Input: part model. Units: mm. Frame: model coordinates. Face numbers are marked on the shaded views. A direction names the side the tool comes from. Give positions to 0.01 mm unless a question says otherwise; leave off trailing zeros. Loops run counter-clockwise (first coordinate to the right, second up) from the corner with the lowest first, then second, coordinate; pieces in that order, holes last. Notation, with made-up numbers: (-32.75, -12) - (1.25, -12) arc R17 ccw to (1.25, 0) - close; hole circle Ø9 at (41, 24). An arc over 180 degrees is marked (long way). Answer as a JSON object with one key per item and string values. Group by question number.
(1) Access query for the marked faces 1, 2 and 3. Directions: +Z, -Z, +X, -X, +Y, -Y. A direction counts if a zero-diameter tool reaches every point of the face in a straight line with its end or side. Return the directions, or none.
(2) Material intervals for L1, parallel to Y at x = 0, z = 13; L2, parallel to Z at x = 12.5, y = 2; L3, parallel to Y at x = 8, z = 184.5, sorted ascending.
(3) Section query A-A (z = 174.5). Return loops of the section in (x, y), plus the area to 3 significant figures.
(4) Section query B-B (z = 126). Return loops of the section in (x, y).
(5) Pin query (flat end, axial travel): P1, Ø5, axis at x = 8.5, z = 166, coming from the -Y side; P2, Ø9.5, axis at x = 0, y = 0, coming from the +Z side; P3, Ø5, axis at y = 7, z = 63, coming from the +X side. Return the tip coordinate at first contact, or that it passes through.
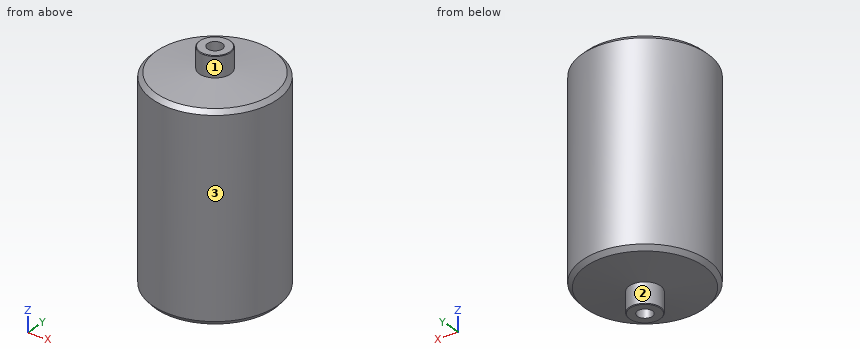
```python
from build123d import *
from OCP.BRepFilletAPI import BRepFilletAPI_MakeChamfer

# Parameters (mm, degrees)
CHAFL_N1_SIZE                     = 3
CHAFL_N1_SIZE2                    = 3.300188603
TALADRO_DE_MARGEN_PARA_M101_D     = 12
TALADRO_DE_MARGEN_PARA_M101_DEPTH = 55.394836286
TALADRO_DE_MARGEN_PARA_M101_TIP   = 3.605163714
TALADRO_DE_MARGEN_PARA_M102_D     = 12
TALADRO_DE_MARGEN_PARA_M102_DEPTH = 55.394836286
TALADRO_DE_MARGEN_PARA_M102_TIP   = 3.605163714
CHAFL_N2_SIZE                     = 0.5


with BuildPart() as part:
    # Croquis1 → Revolución2 (revolve)
    with BuildSketch(Plane(origin=(0, 0, 0), x_dir=(0, 0, -1), z_dir=(1, 0, 0)), mode=Mode.PRIVATE) as revoluci_n2_sk:
        Polygon((0, 0), (0, 12.5), (-16.5, 12.5), (-19.780824882, 50), (-180.219175118, 50), (-183.5, 12.5), (-200, 12.5), (-200, 0), align=None)
    revolve(revoluci_n2_sk.sketch.rotate(Axis((0, 0, 200), (0, 0, -1)), 90), axis=Axis((0, 0, 200), (0, 0, -1)))

    # Chaflán1: one chamfer whose edges measure the first distance from different faces: ONE call of the kernel's chamfer builder (chamfer() names one face for all edges)
    chafl_n1_edges_1 = [part.edges().sort_by_distance(p)[0] for p in [
        (-50, 0, 180.219175118),
    ]]
    chafl_n1_side_1 = [part.faces().sort_by_distance(p)[0] for p in [
        (-50, 0, 100),
    ]]
    chafl_n1_edges_2 = [part.edges().sort_by_distance(p)[0] for p in [
        (-50, 0, 19.780824882),
    ]]
    chafl_n1_side_2 = [part.faces().sort_by_distance(p)[0] for p in [
        (-31.25, 0, 18.140412441),
    ]]
    chafl_n1 = BRepFilletAPI_MakeChamfer(part.part.solid().wrapped)
    for e in chafl_n1_edges_1:
        chafl_n1.Add(CHAFL_N1_SIZE, CHAFL_N1_SIZE2, e.wrapped, chafl_n1_side_1[0].wrapped)  # the first distance lies on this face
    for e in chafl_n1_edges_2:
        chafl_n1.Add(CHAFL_N1_SIZE, CHAFL_N1_SIZE2, e.wrapped, chafl_n1_side_2[0].wrapped)  # the first distance lies on this face
    add(Compound.cast(chafl_n1.Shape()), mode=Mode.REPLACE)

    # Taladro de margen para M101
    with Locations(Plane(origin=(0, 0, 0), x_dir=(-1, 0, 0), z_dir=(0, 0, -1))):
        with Locations((0, 0)):
            Hole(TALADRO_DE_MARGEN_PARA_M101_D / 2, depth=TALADRO_DE_MARGEN_PARA_M101_DEPTH)
            with Locations((0, 0, -(TALADRO_DE_MARGEN_PARA_M101_DEPTH + TALADRO_DE_MARGEN_PARA_M101_TIP / 2))):  # 118° drill point
                Cone(0, TALADRO_DE_MARGEN_PARA_M101_D / 2, TALADRO_DE_MARGEN_PARA_M101_TIP, mode=Mode.SUBTRACT)

    # Taladro de margen para M102
    with Locations(Plane.XY.offset(200)):
        with Locations((0, 0)):
            Hole(TALADRO_DE_MARGEN_PARA_M102_D / 2, depth=TALADRO_DE_MARGEN_PARA_M102_DEPTH)
            with Locations((0, 0, -(TALADRO_DE_MARGEN_PARA_M102_DEPTH + TALADRO_DE_MARGEN_PARA_M102_TIP / 2))):  # 118° drill point
                Cone(0, TALADRO_DE_MARGEN_PARA_M102_D / 2, TALADRO_DE_MARGEN_PARA_M102_TIP, mode=Mode.SUBTRACT)

    # Chaflán2
    chafl_n2_edges = [part.edges().sort_by_distance(p)[0] for p in [
        (-12.5, 0, 200),
        (-12.5, 0, 0),
    ]]
    chamfer(chafl_n2_edges, length=CHAFL_N2_SIZE)


solid = part.part
```
Recorded:
{
 "1": {"face 1": "+Z", "face 2": "-Z", "face 3": "+Z, -Z"},
 "2": {"L1": "y = -12.5 to -6, 6 to 12.5", "L2": "z = 16.51 to 183.49", "L3": "y = -9.6 to 9.6"},
 "3": {"outline": "circle Ø100 at (0, 0); hole circle Ø12 at (0, 0)", "area": "7,740 mm^2"},
 "4": {"outline": "circle Ø100 at (0, 0)"},
 "5": {"P1": "stops at y = -49.64", "P2": "stops at z = 143.85", "P3": "stops at x = 49.8"}
}
